```python
from build123d import *

# Parameters (mm, degrees)
BOSS_EXTRUDE2_DEPTH   = 25
SKETCH6_R             = 4
CUT_EXTRUDE2_DEPTH    = 78.032036302
CUT_EXTRUDE3_DEPTH    = 78.032036302
SKETCH9_R             = 1.5
CUT_EXTRUDE4_DEPTH    = 78.032036302
CROQUIS2_W            = 41
CROQUIS2_H            = 20.5
CORTAR_EXTRUIR1_DEPTH = 10


with BuildPart() as part:
    # Sketch3 → Boss-Extrude2 (new body)
    with BuildSketch(Plane.XY):
        Polygon((-79.925523148, 45.386502584), (-27.042967192, 45.386502584), (-24.925523148, 45.386502584), (-24.925523148, -19.613497416), (-26.925523148, -19.613497416), (-26.925523148, 43.389953837), (-79.925523148, 43.389953837), (-79.925523148, -19.613497416), (-81.925523148, -19.613497416), (-81.925523148, 45.386502584), align=None)
    extrude(amount=BOSS_EXTRUDE2_DEPTH)

    # Sketch6 → Cut-Extrude2 (cut, through all)
    with BuildSketch(Plane.ZY.offset(81.925523148)):
        with Locations(Location((12.5, -5.613497416, 0), (0, 0, 270))):
            Circle(SKETCH6_R)
    extrude(amount=-CUT_EXTRUDE2_DEPTH, mode=Mode.SUBTRACT)

    # Sketch8 → Cut-Extrude3 (cut, through all)
    with BuildSketch(Plane.ZY.offset(81.925523148)):
        with BuildLine():
            Line((0, -19.613497416), (12.5, -19.613497416))
            ThreePointArc((12.5, -19.613497416), (3.661165213, -15.952332159), (0, -7.113497352))
            Line((0, -7.113497352), (0, -19.613497416))
        make_face()
        with BuildLine():
            Line((12.5, -19.613497416), (25, -19.613497416))
            Line((25, -19.613497416), (25, -7.113497416))
            ThreePointArc((25, -7.113497416), (21.338834765, -15.952332181), (12.5, -19.613497416))
        make_face()
    extrude(amount=-CUT_EXTRUDE3_DEPTH, mode=Mode.SUBTRACT)

    # Sketch9 → Cut-Extrude4 (cut, through all)
    with BuildSketch(Plane(origin=(-24.925523148, 0, 0), x_dir=(0, 0, -1), z_dir=(1, 0, 0))):
        with Locations(Location((-12.500000994, 1.386498436, 0), (0, 0, 90))):
            Circle(SKETCH9_R)
        with Locations(Location((-5.500000994, -5.613501564, 0), (0, 0, 90))):
            Circle(SKETCH9_R)
        with Locations(Location((-12.500000994, -12.613501564, 0), (0, 0, 90))):
            Circle(SKETCH9_R)
        with Locations(Location((-19.500000994, -5.613501564, 0), (0, 0, 90))):
            Circle(SKETCH9_R)
    extrude(amount=-CUT_EXTRUDE4_DEPTH, mode=Mode.SUBTRACT)

    # Croquis2 → Cortar-Extruir1 (cut)
    with BuildSketch(Plane(origin=(0, 45.386502584, 0), x_dir=(1, 0, 0), z_dir=(0, 1, 0))):
        with Locations((-53.425523148, -12.5)):
            Rectangle(CROQUIS2_W, CROQUIS2_H)
    extrude(amount=-CORTAR_EXTRUIR1_DEPTH, mode=Mode.SUBTRACT)


solid = part.part
```
Can you work these out from the model? Positions are in its coordinate system, mm. A direction names the side the tool comes from. Coordinates: 2 decimals unless noted, no trailing zeros. Loops run counter-clockwise (first coordinate to the right, second up) from the corner with the lowest first, then second, coordinate; pieces in that order, holes last.
1) Imagine slicing it at A-A on x = -71.5. List the corners of the cut face in (y, z) for me, plus the area to 3 significant figures.
2) Imagine slicing it at D-D on z = 23.75. List the corners of the cut face in (x, y) for me, plus the area to 3 significant figures.
3) Thinking about a two-plate mould opening in Z: for faces 4 (the flat face through (-79.926, 12, 12)), 5 (the cylindrical face through (-25.912, -5.809, 6.987)), 6 (the flat face through (-53, 45, 0)), which applies, pulls with the +Z half, pulls with the -Z half, needs draft (parallel to the pull), parting line crosses it, or undercut?
4) Imagine slicing it at C-C on z = 15.5. List the corners of the cut face in (x, y) for me, plus the area to 3 significant figures.
5) Imagine slicing it at B-B on y = 34. List the corners of the cut face in (x, z) for me, plus the area to 3 significant figures.
6) I need wall thicknesses on probe 1 along X at (y, z) = (41, 1.5); probe 2 along Y at (x, z) = (-78, 9.5). Which ranges of each line are inside material? Lowest first, please.
7) Which directions (+Z, -Z, +X, -X, +Y, -Y) give clear straight access to the entire face, cutting with the end or side of a thin tool? Please do faces 1 (the cylindrical face through (-25.912, 1.191, 13.987)), 2 (the flat face through (-54, 44, 22.75)), 3 (the flat face through (-26.926, 11, 12)).
8) For pin 1 (2.5 mm diameter, centred on y = -5.61, z = 19.5, fed in from -X), with a flat end and sliding along its axis, tell me the tip position at first contact or that it passes through.
Completed:
1. outline: (43.39, 0) - (45.39, 0) - (45.39, 2.25) - (43.39, 2.25) - close; (43.39, 22.75) - (45.39, 22.75) - (45.39, 25) - (43.39, 25) - close
1. area: 8.98 mm2
2. outline: (-81.93, -12.56) - (-79.93, -12.56) - (-79.93, 43.39) - (-26.93, 43.39) - (-26.93, -12.56) - (-24.93, -12.56) - (-24.93, 45.39) - (-81.93, 45.39) - close
2. area: 338 mm2
3. face 4: needs draft
3. face 5: undercut
3. face 6: pulls with the -Z half
4. outline: (-81.93, -19.25) - (-79.93, -19.25) - (-79.93, -8.26) - (-81.93, -8.26) - close; (-81.93, -2.97) - (-79.93, -2.97) - (-79.93, 43.39) - (-73.93, 43.39) - (-73.93, 45.39) - (-81.93, 45.39) - close; (-32.93, 43.39) - (-26.93, 43.39) - (-26.93, -2.97) - (-24.93, -2.97) - (-24.93, 45.39) - (-32.93, 45.39) - close; (-26.93, -19.25) - (-24.93, -19.25) - (-24.93, -8.26) - (-26.93, -8.26) - close
4. area: 261 mm2
5. outline: (-81.93, 0) - (-79.93, 0) - (-79.93, 25) - (-81.93, 25) - close; (-26.93, 0) - (-24.93, 0) - (-24.93, 25) - (-26.93, 25) - close
5. area: 100 mm2
6. probe 1: x = -81.93 to -79.93, -26.93 to -24.93
6. probe 2: y = 43.39 to 45.39
7. face 1: +X, -X
7. face 2: +Y, -Y
7. face 3: +Z, -Z, -Y
8. pin 1: passes through
